Work out the finished part from the listing and answer in its coordinate system (mm). Round coordinates to 2 decimals unless told otherwise and drop trailing zeros. Order: outer loops, then holes, each group sorted by start corner. A loop starts at its lowest first (then second) coordinate and runs counter-clockwise, first axis right, second up. Notation, with made-up numbers: (-5.5, 10) - (41.5, 10) arc R18 cw to (41.5, 28) - close; hole circle Ø9 at (58.25, 78). An arc over 180 degrees is marked (long way). Use one line per item in the form item = value. Start each with the question number.
Q1. The part is cut by section B-B on z = 7. Determine the outline of the cut face in (x, y), plus the area to 3 significant figures.
Q2. The part is cut by section A-A on z = 3.25. Determine the outline of the cut face in (x, y), plus the area to 3 significant figures.
Q3. Given P1, Ø5, axis at y = 15, z = 2.5, coming from the +X side; P2, Ø2, axis at x = -11.5, z = 6, coming from the +Y side, each flat-ended and moving along its own axis, determine where each tip first touches the part or whether it passes through.
Q4. Find the intervals of material crossed by line 1 (Y direction, x = 8, z = 4.75); line 2 (X direction, y = -8, z = 4.5); line 3 (X direction, y = -2, z = 8.25), in increasing order. Write a range as [from, to].
from build123d import *

# Parameters (mm, degrees)
F2_R     = 4.2022748897
F4_R     = 4
F5_DEPTH = 25
F6_DEPTH = 25


# Not quite as in the source:
# - the program builds the solid bodies; features that only make, move or delete a surface that nothing else refers to are left out


with BuildPart() as f3:
    # F2 (on Front) → F3 (revolve)
    with BuildSketch(Plane.XZ):
        with Locations((-15, 5)):
            Circle(F2_R)
    revolve(axis=Axis((0, 0, 2.5), (0, 0, -1)))

    # F4 (on Top) → F5 (cut)
    with BuildSketch(Plane.XY):
        with Locations((-10.4587538705, 18.2102846621)):
            Circle(F4_R)
    extrude(amount=F5_DEPTH, mode=Mode.SUBTRACT)

    # F4 (on Top) → F6 (cut)
    with BuildSketch(Plane.XY):
        with Locations((-10.4587538705, 18.2102846621)):
            Circle(F4_R)
    extrude(amount=F6_DEPTH, mode=Mode.SUBTRACT)


solid = f3.part
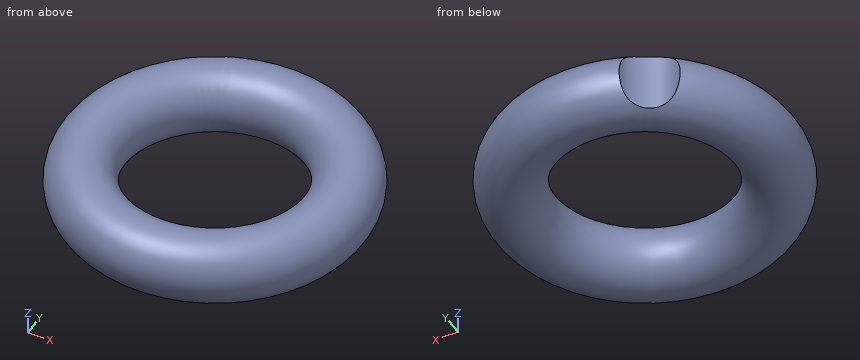
Found:
q1.outline = (-11.85, 14.46) arc R18.7 ccw (long way) to (-6.52, 17.52) arc R4 cw to start; hole circle Ø22.61 at (0, 0)
q1.area = 689 mm²
q2.outline = (-11.98, 14.51) arc R18.82 ccw (long way) to (-6.5, 17.66) arc R4 cw to start; hole circle Ø22.36 at (0, 0)
q2.area = 712 mm²
q3.P1 = 14.03
q3.P2 = 14.68
q4.line_1 = [-17.45, -7.26], [7.26, 17.45]
q4.line_2 = [-17.42, -7.3], [7.3, 17.42]
q4.line_3 = [-17.55, -12.17], [12.17, 17.55]
